Geometry: see drawing. Coordinates: mm, zero at the bounding-box minimum. A direction names the side the tool comes from. Round coordinates to 2 decimals unless told otherwise and drop trailing zeros. Order: outer loops, then holes, each group sorted by start corner. A loop starts at its lowest first (then second) coordinate and runs counter-clockwise, first axis right, second up. Notation, with made-up numbers: (60, -4) -> (101, -4) arc R14 cw to (101, 15) -> close; hole circle Ø10 at (86, -31). An arc over 180 degrees is marked (long way). Put each result on its own line as item: value.
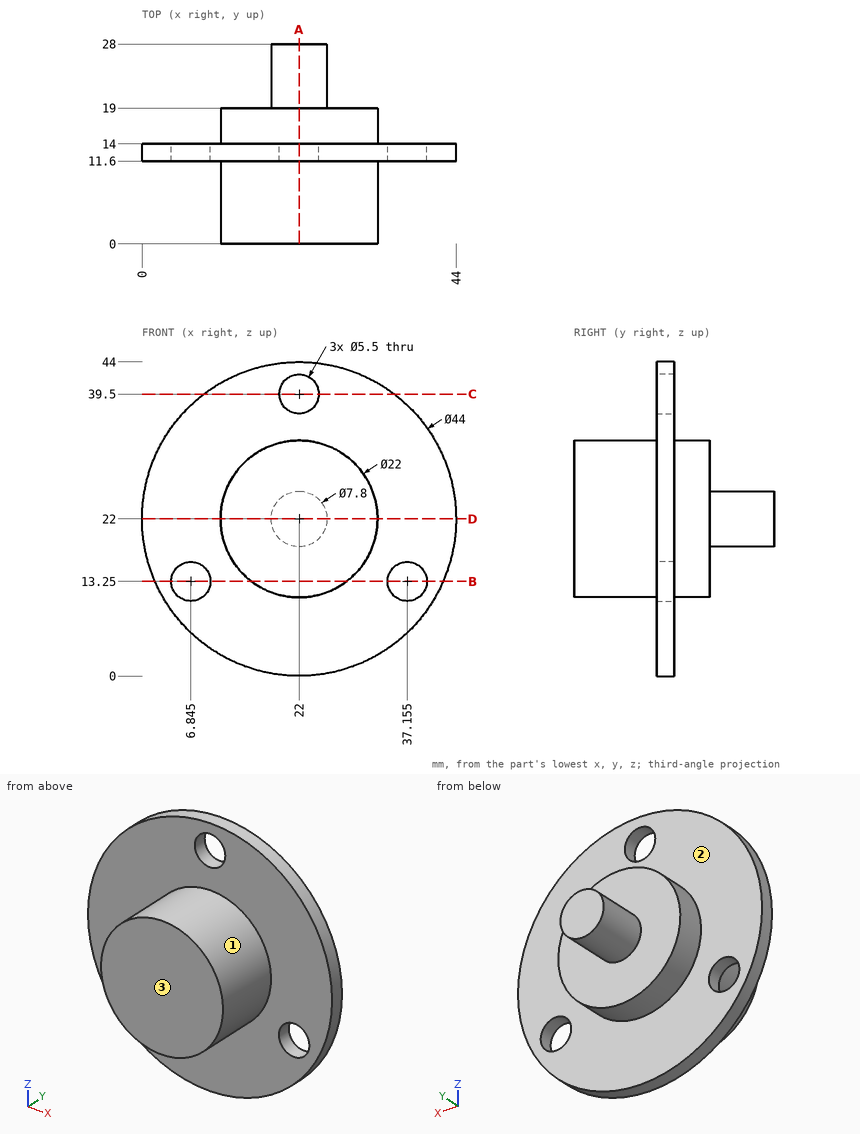
1. Cut plane B-B on z = 13.25. Return loops of the section in (x, y) (1 decimal), and give its area (3 significant figures).
Ans:
outline: (1.8, 11.6) -> (4.1, 11.6) -> (4.1, 14) -> (1.8, 14) -> close; (9.6, 11.6) -> (15.3, 11.6) -> (15.3, 0) -> (28.7, 0) -> (28.7, 11.6) -> (34.4, 11.6) -> (34.4, 14) -> (28.7, 14) -> (28.7, 19) -> (15.3, 19) -> (15.3, 14) -> (9.6, 14) -> close; (39.9, 11.6) -> (42.2, 11.6) -> (42.2, 14) -> (39.9, 14) -> close
area: 292 mm²
2. Contact query for flat-ended pins moving along their axis: P1, Ø6, axis at x = 16, y = 6.5, coming from the +Z side; P2, Ø9, axis at x = 6.84, z = 13.25, coming from the +Y side; P3, Ø10, axis at x = 30, y = 12, coming from the +Z side (1 decimal). Output: stop coordinate, or through.
Ans:
P1: z = 32.58
P2: y = 14
P3: z = 43.8
3. Cut plane D-D on z = 22. Return loops of the section in (x, y).
Ans:
outline: (0, 11.6) -> (11, 11.6) -> (11, 0) -> (33, 0) -> (33, 11.6) -> (44, 11.6) -> (44, 14) -> (33, 14) -> (33, 19) -> (25.9, 19) -> (25.9, 28) -> (18.1, 28) -> (18.1, 19) -> (11, 19) -> (11, 14) -> (0, 14) -> close
4. Set-up query: the marked faces 1, 2 and 3. Return all of +Z, -Z, +X, -X, +Y, -Y with unobstructed straight access to the full face (end or side cutting, diameter ignored); none if empty.
Ans:
face 1: -Y
face 2: +Y
face 3: +Z, -Z, +X, -X, -Y
5. Material intervals for probe 1 along X at (y, z) = (12.5, 13.25) (1 decimal); probe 2 along Z at (x, y) = (38, 13.5) (1 decimal); probe 3 along Y at (x, z) = (27, 4), sorted ascending.
Ans:
probe 1: 1.8 to 4.1, 9.6 to 34.4, 39.9 to 42.2
probe 2: 6.9 to 10.6, 15.9 to 37.1
probe 3: 11.6 to 14
6. Cut plane C-C on z = 39.5. Return loops of the section in (x, y).
Ans:
outline: (8.67, 11.6) -> (19.25, 11.6) -> (19.25, 14) -> (8.67, 14) -> close; (24.75, 11.6) -> (35.33, 11.6) -> (35.33, 14) -> (24.75, 14) -> close
7. Cut plane A-A on x = 22. Return loops of the section in (y, z).
Ans:
outline: (0, 11) -> (11.6, 11) -> (11.6, 0) -> (14, 0) -> (14, 11) -> (19, 11) -> (19, 18.1) -> (28, 18.1) -> (28, 25.9) -> (19, 25.9) -> (19, 33) -> (14, 33) -> (14, 36.75) -> (11.6, 36.75) -> (11.6, 33) -> (0, 33) -> close; (11.6, 42.25) -> (14, 42.25) -> (14, 44) -> (11.6, 44) -> close
